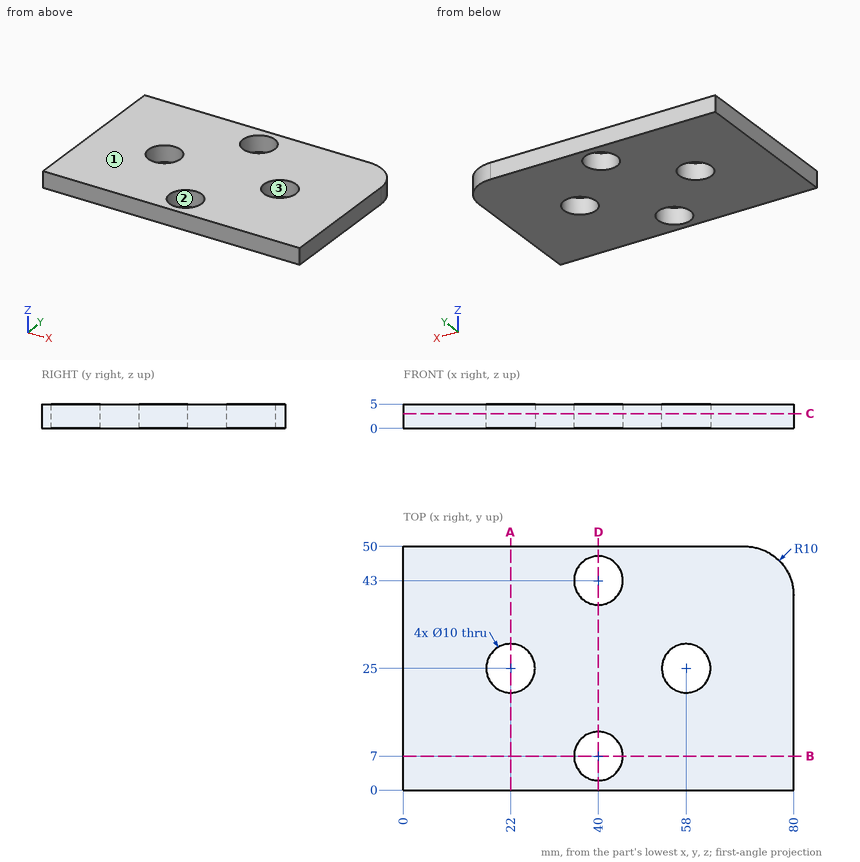
Could you check a few things on this drawing? It's one solid part, dimensions in mm from its lowest x, y, z. Round coordinates to 2 decimals unless told otherwise and drop trailing zeros. Order: outer loops, then holes, each group sorted by start corner. A loop starts at its lowest first (then second) coordinate and runs counter-clockwise, first axis right, second up. Notation, with made-up numbers: M 24,-10.5 L 61,-10.5 A24 cw 61,24.5 Z; hole C 2.5,70.25 d5. An arc over 180 degrees is marked long. Use a Markdown table: item, result.
1) Imagine slicing it at A-A (x = 22). List the corners of the cut face in (y, z) for me.
Geometry says:
| item | result |
|---|---|
| outline | M 0,0 L 20,0 L 20,5 L 0,5 Z; M 30,0 L 50,0 L 50,5 L 30,5 Z |
2) If I drill on line 1 along Y through (x, z) = (40, 2.4); line 2 along Y through (x, z) = (22, 1.7); line 3 along Y through (x, z) = (36.5, 3.45), over which ranges is the centre line in solid material (lowest first)?
Geometry says:
| item | result |
|---|---|
| line 1 | y = 0 to 2, 12 to 38, 48 to 50 |
| line 2 | y = 0 to 20, 30 to 50 |
| line 3 | y = 0 to 3.43, 10.57 to 39.43, 46.57 to 50 |
3) If we mould it in two halves opening along X, with no side actions, what happens to the marked faces 1, 2 and 3? For each: +X half, -X half, draft (parallel to the pull), parting line (faces both ways), or undercut.
Geometry says:
| item | result |
|---|---|
| face 1 | draft |
| face 2 | undercut |
| face 3 | undercut |
4) Imagine slicing it at C-C (z = 3). List the corners of the cut face in (x, y) for me, then the cut area to 3 significant figures.
Geometry says:
| item | result |
|---|---|
| outline | M 0,0 L 80,0 L 80,40 A10 ccw 70,50 L 0,50 Z; hole C 22,25 d10; hole C 40,7 d10; hole C 40,43 d10; hole C 58,25 d10 |
| area | 3,660 mm² |
5) Imagine slicing it at D-D (x = 40). List the corners of the cut face in (y, z) for me.
Geometry says:
| item | result |
|---|---|
| outline | M 0,0 L 2,0 L 2,5 L 0,5 Z; M 12,0 L 38,0 L 38,5 L 12,5 Z; M 48,0 L 50,0 L 50,5 L 48,5 Z |
6) Imagine slicing it at B-B (y = 7). List the corners of the cut face in (x, z) for me, then the cut area to 3 significant figures.
Geometry says:
| item | result |
|---|---|
| outline | M 0,0 L 35,0 L 35,5 L 0,5 Z; M 45,0 L 80,0 L 80,5 L 45,5 Z |
| area | 350 mm² |
7) I'm going to push flat-ended pins straight in: P1, Ø3, axis at x = 47.5, y = 32, coming from the -Z side; P2, Ø9, axis at x = 40, y = 43, coming from the -Z side. Where does each tip first touch, or does it pass through?
Geometry says:
| item | result |
|---|---|
| P1 | stops at z = 0 |
| P2 | passes through |
